Autodesk Inventor part; units mm, degrees
ref_plane "FDT_KSAUFSATZ_XY" through (0, 0, 20) normal (0, 0, 1) x (-1, 0, 0)
ref_plane "FDT_KSAUFSATZ_YZ" through (0, 0, 20) normal (-1, 0, 0) x (0, -1, 0)
ref_plane "FDT_KSAUFSATZ_ZX" through (0, 0, 20) normal (0, -1, 0) x (0, 0, 1)
sketch "Sketch_2" plane through (0, 0, 0) normal (1, 0, 0) x (0, 1, 0)
  line L0 (0, -377) -> (0, 9)
  line L1 (0, 9) -> (8, 9)
  line L2 (8, 9) -> (8, -367)
  line L3 (8, -367) -> (20, -367)
  line L4 (20, -367) -> (20, -377)
  line L5 (20, -377) -> (0, -377)
  line L6 (0, -377) -> (0, 9)
revolve "Revolution1" add sketch "Sketch_2" angle 360 about axis through (0, 0, -377) along (0, 0, -1)
sketch "Sketch_6" plane through (0, 0, 0) normal (1, 0, 0) x (0, 1, 0)
  line L0 (0, 8) -> (0, 33)
  line L1 (0, 33) -> (5.233, 33)
  line L2 (5.233, 33) -> (6, 32.233)
  line L3 (6, 32.233) -> (6, 12.9727)
  line L4 (6, 12.9727) -> (5.1362, 10.5994)
  arc A0 (5.1362, 10.5994) -> (5.1, 10.3942) centre (5.7, 10.3942) ccw
  line L5 (5.1, 10.3942) -> (5.1, 9.6)
  arc A1 (5.1, 9.6) -> (5.7, 9) centre (5.7, 9.6) ccw
  line L6 (5.7, 9) -> (6, 9)
  line L7 (6, 9) -> (6, 8)
  line L8 (6, 8) -> (0, 8)
  line L9 (0, 8) -> (0, 33)
revolve "Revolution2" add sketch "Sketch_6" angle 360 about axis through (0, 0, 8) along (0, 0, -1)
thread "Thread1"
sketch "Sketch_7" plane through (0, 0, 2.5) normal (0, 0, 1) x (1, 0, 0)
  line L0 (-13, 26) -> (-13, -13)
  line L1 (-13, -13) -> (-6.5, -13)
  line L2 (-6.5, -13) -> (-6.5, 13)
  line L3 (-6.5, 13) -> (6.5, 13)
  line L4 (6.5, 13) -> (6.5, -13)
  line L5 (6.5, -13) -> (13, -13)
  line L6 (13, -13) -> (13, 26)
  line L7 (13, 26) -> (-13, 26)
extrude "Extrusion1" cut sketch "Sketch_7" along normal blind 7.5
ref_plane "FDT_KSAUFSATZ_XY" through (0, 0, 20) normal (0, 0, 1) x (-1, 0, 0)
ref_plane "FDT_KSAUFSATZ_YZ" through (0, 0, 20) normal (-1, 0, 0) x (0, -1, 0)
ref_plane "FDT_KSAUFSATZ_ZX" through (0, 0, 20) normal (0, -1, 0) x (0, 0, 1)
ref_plane "FDT_NUT_XY" through (0, 0, 20) normal (0, 0, 1) x (-1, 0, 0)
ref_plane "FDT_NUT_YZ" through (0, 0, 20) normal (-1, 0, 0) x (0, -1, 0)
ref_plane "FDT_NUT_ZX" through (0, 0, 20) normal (0, -1, 0) x (0, 0, 1)
ref_plane "KS_XY" through (0, 0, 0) normal (0, 0, -1) x (1, 0, 0)
ref_plane "KS_YZ" through (0, 0, 0) normal (1, 0, 0) x (0, -1, 0)
ref_plane "KS_ZX" through (0, 0, 0) normal (0, -1, 0) x (0, 0, -1)
ref_plane "NUT1_XY" through (0, 0, 24) normal (0, 0, 1) x (1, 0, 0)
ref_plane "NUT1_YZ" through (0, 0, 24) normal (1, 0, 0) x (0, 1, 0)
ref_plane "NUT1_ZX" through (0, 0, 24) normal (0, 1, 0) x (0, 0, 1)
properties part number "193993 DSNU-40-300-P---(A---00--0-KS)"
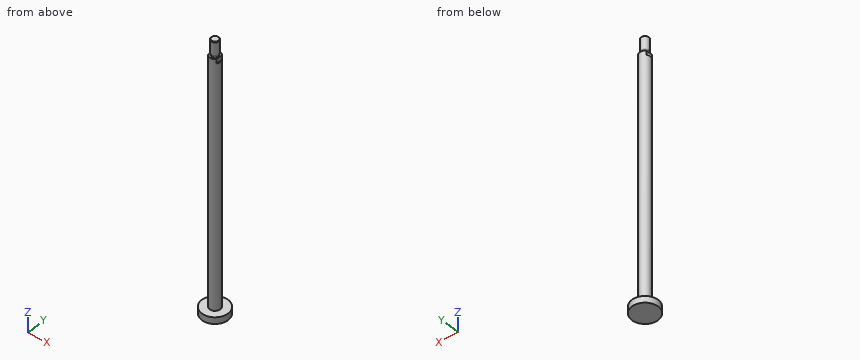
Geometry check sheet. Reference: the model listing, model coordinates, mm. Round coordinates to 2 decimals unless told otherwise and drop trailing zeros. Loops run counter-clockwise (first coordinate to the right, second up) from the corner with the lowest first, then second, coordinate; pieces in that order, holes last. Notation, with made-up numbers: (-17.75, -5) -> (-12.75, -5) arc R26 ccw to (-12.75, 17) -> close; hole circle Ø8 at (79, 12.5). An arc over 180 degrees is marked (long way). Answer as a JSON object with one key per item and string values. Group by question number.
Item 1: Cross-section at A-A, the plane y = 0. Record the cut outline in (x, z).
Item 2: Cross-section at B-B, the plane z = -76.5. Record the cut outline in (x, y), plus the area to 3 significant figures.
Item 3: Thickness scan on line 1 along Z through (x, y) = (-4.5, -9); line 2 along X through (y, z) = (-6, -222). Record the ranges inside material, lowest first.
Item 4: Depth check by flat-ended pin: pin 1 Ø1 at (x, z) = (2, -107) entering from -Y; pin 2 Ø7 at (y, z) = (1.5, 7) entering from -X; pin 3 Ø1.2 at (x, y) = (7, 1.5) entering from +Z; pin 4 Ø6 at (y, z) = (12, -243.5) entering from -X. Enter the tip coordinate at first touch or a pass-through.
Item 5: Cross-section at C-C, the plane x = -15. Record the cut outline in (y, z), plus the area to 3 significant figures.
Determined:
{
 "1": {"outline": "(-20, -377) -> (20, -377) -> (20, -367) -> (8, -367) -> (8, 2.5) -> (6.5, 2.5) -> (6.5, 9) -> (5.7, 9) arc R0.6 cw to (5.1, 9.6) -> (5.1, 10.39) arc R0.6 cw to (5.14, 10.6) -> (6, 12.97) -> (6, 32.23) -> (5.23, 33) -> (-5.23, 33) -> (-6, 32.23) -> (-6, 12.97) -> (-5.14, 10.6) arc R0.6 cw to (-5.1, 10.39) -> (-5.1, 9.6) arc R0.6 cw to (-5.7, 9) -> (-6.5, 9) -> (-6.5, 2.5) -> (-8, 2.5) -> (-8, -367) -> (-20, -367) -> close"},
 "2": {"outline": "circle Ø16 at (0, 0)", "area": "201 mm²"},
 "3": {"line 1": "z = -377 to -367", "line 2": "x = -5.29 to 5.29"},
 "4": {"pin 1": "stops at y = -7.86", "pin 2": "stops at x = -6.5", "pin 3": "stops at z = 9", "pin 4": "passes through"},
 "5": {"outline": "(-13.23, -377) -> (13.23, -377) -> (13.23, -367) -> (-13.23, -367) -> close", "area": "265 mm²"}
}
